Autodesk Inventor part; units mm, degrees
ref_plane "YZ Plane" through (0, 0, 0) normal (1, 0, 0) x (0, 1, 0)
ref_plane "XZ Plane" through (0, 0, 0) normal (0, 1, 0) x (-1, 0, 0)
ref_plane "XY Plane" through (0, 0, 0) normal (0, 0, 1) x (1, 0, 0)
sketch "Sketch1" plane through (0, 0, 0) normal (0, 1, 0) x (-1, 0, 0)
  line L0 (0, 0) -> (101.6, 0)
  line L1 (101.6, 0) -> (101.6, 50.8)
  line L2 (101.6, 50.8) -> (0, 50.8)
  line L3 (0, 50.8) -> (0, 0)
  line L4 (101.6, 0) -> (28.575, 0)
  line L5 (28.575, 0) -> (28.575, 50.8)
  line L6 (28.575, 50.8) -> (101.6, 50.8)
  line L7 (101.6, 50.8) -> (101.6, 0)
  line L8 (28.575, 0) -> (0, 0)
  line L9 (0, 0) -> (0, 12.7)
  line L10 (0, 12.7) -> (28.575, 12.7)
  line L11 (28.575, 12.7) -> (28.575, 0)
  line L12 (28.575, 50.8) -> (0, 50.8)
  line L13 (0, 50.8) -> (0, 38.1)
  line L14 (0, 38.1) -> (28.575, 38.1)
  line L15 (28.575, 38.1) -> (28.575, 50.8)
  line L16 (96.8375, 0) -> (84.1375, 0)
  line L17 (84.1375, 0) -> (84.1375, 3.175)
  line L18 (84.1375, 3.175) -> (96.8375, 3.175)
  line L19 (96.8375, 3.175) -> (96.8375, 0)
  line L20 (71.4375, 0) -> (58.7375, 0)
  line L21 (58.7375, 0) -> (58.7375, 3.175)
  line L22 (58.7375, 3.175) -> (71.4375, 3.175)
  line L23 (71.4375, 3.175) -> (71.4375, 0)
  line L24 (46.0375, 0) -> (33.3375, 0)
  line L25 (33.3375, 0) -> (33.3375, 3.175)
  line L26 (33.3375, 3.175) -> (46.0375, 3.175)
  line L27 (46.0375, 3.175) -> (46.0375, 0)
  line L28 (96.8375, 50.8) -> (84.1375, 50.8)
  line L29 (84.1375, 50.8) -> (84.1375, 47.625)
  line L30 (84.1375, 47.625) -> (96.8375, 47.625)
  line L31 (96.8375, 47.625) -> (96.8375, 50.8)
  line L32 (71.4375, 50.8) -> (58.7375, 50.8)
  line L33 (58.7375, 50.8) -> (58.7375, 47.625)
  line L34 (58.7375, 47.625) -> (71.4375, 47.625)
  line L35 (71.4375, 47.625) -> (71.4375, 50.8)
  line L36 (101.6, 38.1) -> (98.425, 38.1)
  line L37 (98.425, 38.1) -> (98.425, 31.75)
  line L38 (98.425, 31.75) -> (101.6, 31.75)
  line L39 (101.6, 31.75) -> (101.6, 38.1)
  line L40 (101.6, 19.05) -> (98.425, 19.05)
  line L41 (98.425, 19.05) -> (98.425, 12.7)
  line L42 (98.425, 12.7) -> (101.6, 12.7)
  line L43 (101.6, 12.7) -> (101.6, 19.05)
  line L44 (46.0375, 50.8) -> (46.0375, 47.625)
  line L45 (46.0375, 47.625) -> (33.3375, 47.625)
  line L46 (33.3375, 47.625) -> (33.3375, 50.8)
  line L47 (33.3375, 50.8) -> (46.0375, 50.8)
  line L48 (52.3875, 0) -> (77.7875, 0)
  line L49 (77.7875, 0) -> (77.7875, -19.05)
  line L50 (77.7875, -19.05) -> (52.3875, -19.05)
  line L51 (52.3875, -19.05) -> (52.3875, 0)
  line L52 (52.3875, 50.8) -> (52.3875, 69.85)
  line L53 (52.3875, 69.85) -> (77.7875, 69.85)
  line L54 (77.7875, 69.85) -> (77.7875, 50.8)
  line L55 (77.7875, 50.8) -> (52.3875, 50.8)
  circle A0 centre (65.0875, -9.525) radius 3.302
  circle A1 centre (65.0875, 60.325) radius 3.302
  point P0 (96.8375, 0)
  point P1 (96.8375, 50.8)
  point P2 (84.1375, 50.8)
  point P3 (71.4375, 50.8)
  point P4 (58.7375, 50.8)
  point P5 (46.0375, 50.8)
  point P6 (33.3375, 50.8)
  point P7 (33.3375, 0)
  point P8 (46.0375, 0)
  point P9 (58.7375, 0)
  point P10 (71.4375, 0)
  point P11 (84.1375, 0)
  dimension "d56" = 101.6
  dimension "d57" = 50.8
  dimension "d58" = 73.025
  dimension "d59" = 50.8
  dimension "d60" = 12.7
  dimension "d61" = 12.7
  dimension "d62" = 12.7
  dimension "d63" = 3.175
  dimension "d64" = 12.7
  dimension "d65" = 3.175
  dimension "d66" = 12.7
  dimension "d67" = 4.7625
  dimension "d68" = 12.7
  dimension "d69" = 3.175
  dimension "d70" = 12.7
  dimension "d71" = 12.7
  dimension "d72" = 3.175
  dimension "d73" = 12.7
  dimension "d74" = 3.175
  dimension "d77" = 4.7625
  dimension "d78" = 12.7
  dimension "d79" = 3.175
  dimension "d80" = 6.35
  dimension "d81" = 12.7
  dimension "d82" = 3.175
  dimension "d83" = 6.35
  dimension "d84" = 12.7
  dimension "d86" = 44.45
  dimension "d89" = 3.175
  dimension "d90" = 12.7
  dimension "d91" = 12.7
  dimension "d94" = 25.4
  dimension "d96" = 23.8125
  dimension "d97" = 23.8125
  dimension "d99" = 25.4
  dimension "d116" = 6.604
  dimension "d117" = 9.525
  dimension "d118" = 6.604
  dimension "d119" = 9.525
  dimension "d122" = 9.525
  dimension "d123" = 9.525
extrude "Extrusion4" add sketch "Sketch1" along normal blind 12.7 contours L5 L2 L46 L45 L44 L33 L34 L35 L29 L30 L31 L1 L36 L37 L38 L40 L41 L42 L0 L19 L18 L17 L23 L22 L21 L27 L26 L25 | L3 L14 L5 L10 | L0 L49 L50 L51 | L52 L53 L54 L2
equation "\"d124\" = d78"
equation "\"BendRadius\" = Thickness"
equation "\"BendReliefWidth\" = Thickness"
equation "\"BendReliefDepth\" = 0.5 * Thickness"
equation "\"CornerReliefSize\" = 4 * Thickness"
equation "\"MinimumRemnant\" = 2 * Thickness"
equation "\"TransitionRadius\" = BendRadius"
equation "\"JacobiRadiusSize\" = BendRadius"
equation "\"GapSize\" = Thickness"
properties part number "Burrow_Base_Detachable_EXT"
Source: CAD feature listing. Evaluate the final solid. Frame: model axes, mm. A direction names the side the tool comes from. Round coordinates to 2 decimals unless told otherwise and drop trailing zeros. Loops run counter-clockwise (first coordinate to the right, second up) from the corner with the lowest first, then second, coordinate; pieces in that order, holes last. Notation, with made-up numbers: M -19,88 L -3,88 A13 ccw -3,103 Z; hole C -26.5,85.5 d1. An arc over 180 degrees is marked long. Return JSON: item names as keys, results as strings. Group by question number.
1. Mould query, pull axis Z, two halves, no side actions, for faces 5 (the face through (-61.79, 6.26, -9.67)), 6 (the face through (0, 6, 26)), 7 (the face through (-81, 6, 50.8)), 8 (the face through (-40, 6, 3.175)). Classes: released by +Z, released by -Z, zero draft, split by the parting line, or undercut.
2. Reachability of faces 1 (the face through (-98.425, 6, 16)), 2 (the face through (-52.388, 6, 60)), 3 (the face through (-58.738, 6, 2)), 4 (the face through (-90, 6, 47.625)) from +Z, -Z, +X, -X, +Y, -Y: full face, straight path, thin tool, end or side. Return the list, or none.
3. Pin query (flat end, axial travel): pin 1 (4 mm diameter, centred on x = -74, z = 29, fed in from -Y); pin 2 (4 mm diameter, centred on y = 8, z = 63, fed in from -X); pin 3 (3 mm diameter, centred on x = -79.5, y = 4, fed in from -Z); pin 4 (6 mm diameter, centred on y = 9.5, z = 1, fed in from +X) (3 decimals). Return the tip coordinate at first contact, or that it passes through.
4. Section query C-C on y = 3.5. State how many separate pieces and enclosed holes the cut face has, and give its area (3 significant figures).
5. Section query A-A on x = -11. Output: boundary loops of the cut face in (y, z), and give its area (3 significant figures).
6. Material intervals for line 1 along X through (y, z) = (11.5, 48) (1 decimal); line 2 along X through (y, z) = (5.5, -2); line 3 along Z through (x, y) = (-27, 11.75), sorted ascending. Write a range as from..to.
7. Section query B-B on z = 41. Output: boundary loops of the cut face in (x, y) (3 decimals).
Checks:
{
 "1": {"face 5": "undercut", "face 6": "zero draft", "face 7": "released by +Z", "face 8": "released by -Z"},
 "2": {"face 1": "-X, +Y, -Y", "face 2": "+Z, +X, +Y, -Y", "face 3": "+Y, -Y", "face 4": "+Z, +Y, -Y"},
 "3": {"pin 1": "stops at y = 0", "pin 2": "stops at x = -77.79", "pin 3": "stops at z = 0", "pin 4": "stops at x = -28.575"},
 "4": {"separate pieces": "1", "enclosed holes": "4", "area": "5,050 mm²"},
 "5": {"outline": "M 0,12.7 L 12.7,12.7 L 12.7,38.1 L 0,38.1 Z", "area": "323 mm²"},
 "6": {"line 1": "x = -101.6..-96.8, -84.1..-71.4, -58.7..-46, -33.3..-28.6", "line 2": "x = -77.79..-52.39", "line 3": "z = 12.7..38.1"},
 "7": {"outline": "M -101.6,0 L -28.575,0 L -28.575,12.7 L -101.6,12.7 Z"}
}
